from build123d import *

# Parameters (mm, degrees)
SKETCH1_R                                         = 42.9895
SKETCH1_R_2                                       = 36.6395
BOSS_EXTRUDE1_DEPTH                               = 19.05
BOSS_EXTRUDE2_DEPTH                               = 19.05
FILLET1_R                                         = 12.7
CHAMFER1_SIZE                                     = 1.5875
CSK_FOR_8_FLAT_HEAD_MACHINE_SCREW_100_D           = 4.9149
CSK_FOR_8_FLAT_HEAD_MACHINE_SCREW_100_CSINK_D     = 8.4328
CSK_FOR_8_FLAT_HEAD_MACHINE_SCREW_100_CSINK_ANGLE = 100


with BuildPart() as part:
    # Sketch1 → Boss-Extrude1 (new body)
    with BuildSketch(Plane.XY):
        with Locations(Location((0, 0, 0), (0, 0, 180))):
            Circle(SKETCH1_R)
        with Locations(Location((0, 0, 0), (0, 0, 180))):
            Circle(SKETCH1_R_2, mode=Mode.SUBTRACT)
    extrude(amount=BOSS_EXTRUDE1_DEPTH)

    # Sketch3 → Boss-Extrude2 (add, through all)
    with BuildSketch(Plane.XY.offset(19.05)):
        with BuildLine():
            Line((-6.35, 57.593182132), (-12.321797405, 41.18580361))
            ThreePointArc((-12.321797405, 41.18580361), (0, 42.926029516), (12.321797405, 41.18580361))
            Line((12.321797405, 41.18580361), (6.35, 57.593182132))
            ThreePointArc((6.35, 57.593182132), (3.875959319, 60.817414721), (0, 62.0395))
            ThreePointArc((0, 62.0395), (-3.875959319, 60.817414721), (-6.35, 57.593182132))
        make_face()
    extrude(amount=-BOSS_EXTRUDE2_DEPTH)

    # Fillet1
    fillet1_edges = [part.edges().sort_by_distance(p)[0] for p in [
        (12.321797405, 41.18580361, 9.525),
        (-12.321797405, 41.18580361, 9.525),
    ]]
    fillet(fillet1_edges, radius=FILLET1_R)

    # Chamfer1
    chamfer1_edges = [part.edges().sort_by_distance(p)[0] for p in [
        (0, 62.0395, 0),
        (-8.330591024, 52.151553016, 0),
        (-8.330591024, 52.151553016, 19.05),
        (0, 62.0395, 19.05),
        (0, -42.9895, 0),
        (0, -42.9895, 19.05),
        (8.330591024, 52.151553016, 19.05),
        (8.330591024, 52.151553016, 0),
        (12.991632469, 42.355301831, 19.05),
        (12.991632469, 42.355301831, 0),
        (-12.991632469, 42.355301831, 19.05),
        (-12.991632469, 42.355301831, 0),
    ]]
    chamfer(chamfer1_edges, length=CHAMFER1_SIZE)

    # CSK for #8 Flat Head Machine Screw (100)1 (through all)
    with Locations(Plane.XY.offset(19.05)):
        with Locations((0, 55.281971145)):
            CounterSinkHole(CSK_FOR_8_FLAT_HEAD_MACHINE_SCREW_100_D / 2, CSK_FOR_8_FLAT_HEAD_MACHINE_SCREW_100_CSINK_D / 2, counter_sink_angle=CSK_FOR_8_FLAT_HEAD_MACHINE_SCREW_100_CSINK_ANGLE)


solid = part.part
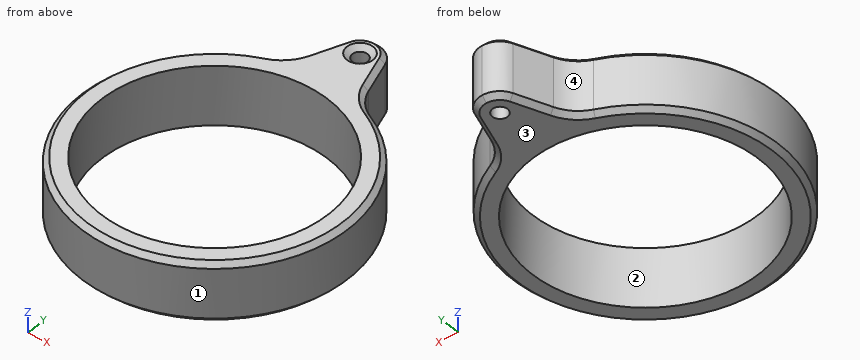
Geometry check sheet. Reference: the model listing, model coordinates, mm. Face numbers are marked on the shaded views. Round coordinates to 2 decimals unless told otherwise and drop trailing zeros. Loops run counter-clockwise (first coordinate to the right, second up) from the corner with the lowest first, then second, coordinate; pieces in that order, holes last.
Item 1: Cross-section at B-B on z = 4. Record the boundary of the cut face in (x, y), then the cut area to 3 significant figures.
Item 2: Mould release check, pull along X, two halves, no side actions. Record for the marked faces 1, 2, 3 and 4: pulls with the +X half, pulls with the -X half, needs draft (parallel to the pull), parting line crosses it, or undercut.
Item 3: Cross-section at A-A on y = 0. Record the boundary of the cut face in (x, z), then the cut area to 3 significant figures.
Item 4: Thickness scan on line 1 (Y direction, x = 0, z = 14.25); line 2 (X direction, y = -0.5, z = 7.25); line 3 (Y direction, x = -2, z = 12.5). Record the ranges inside material, lowest first.
Item 5: Gauge pin test, flat ends, axial feed: pin 1 (6 mm diameter, centred on x = -29, z = 3, fed in from +Y); pin 2 (6 mm diameter, centred on y = 11, z = 15, fed in from -X); pin 3 (10 mm diameter, centred on x = 26, z = 10, fed in from +Y). Record the tip position at first contact, or that the pin passes through.
Answer sheet:
1. outline: (-17.17, 39.41) arc R42.99 ccw (long way) to (17.17, 39.41) arc R12.7 cw to (10.31, 46.71) - (6.35, 57.59) arc R6.76 ccw to (-6.35, 57.59) - (-10.31, 46.71) arc R12.7 cw to start; hole circle Ø73.28 at (0, 0); hole circle Ø4.91 at (0, 55.28)
1. area: 1,900 mm2
2. face 1: parting line crosses it
2. face 2: undercut
2. face 3: needs draft
2. face 4: pulls with the -X half
3. outline: (-42.99, 1.59) - (-41.4, 0) - (-36.64, 0) - (-36.64, 19.05) - (-41.4, 19.05) - (-42.99, 17.46) - close; (36.64, 0) - (41.4, 0) - (42.99, 1.59) - (42.99, 17.46) - (41.4, 19.05) - (36.64, 19.05) - close
3. area: 237 mm2
4. line 1: y = -42.99 to -36.64, 36.64 to 52.82, 57.74 to 62.04
4. line 2: x = -42.99 to -36.64, 36.64 to 42.99
4. line 3: y = -42.94 to -36.58, 36.58 to 53.85, 56.71 to 61.74
5. pin 1: stops at y = 34.24
5. pin 2: stops at x = -42.24
5. pin 3: stops at y = 37.51
